from build123d import *

# Parameters (mm, degrees)
BOSS_EXTRUDE1_DEPTH = 5


with BuildPart() as part:
    # Sketch1 → Boss-Extrude1 (new body)
    with BuildSketch(Plane.XY):
        with BuildLine():
            Line((-150, 40), (-71.83, 40))
            Line((-71.83, 40), (-71.83, -40))
            Line((-71.83, -40), (-150, -40))
            Line((-150, -40), (-150, -100))
            ThreePointArc((-150, -100), (-147.071067812, -107.071067812), (-140, -110))
            Line((-140, -110), (140, -110))
            ThreePointArc((140, -110), (147.071067812, -107.071067812), (150, -100))
            Line((150, -100), (150, -40))
            Line((150, -40), (71.83, -40))
            Line((71.83, -40), (71.83, 40))
            Line((71.83, 40), (150, 40))
            Line((150, 40), (150, 100))
            ThreePointArc((150, 100), (147.071067812, 107.071067812), (140, 110))
            Line((140, 110), (-140, 110))
            ThreePointArc((-140, 110), (-147.071067812, 107.071067812), (-150, 100))
            Line((-150, 100), (-150, 40))
        make_face()
    extrude(amount=BOSS_EXTRUDE1_DEPTH)


solid = part.part
Verification items for the finished model (mm, model axes). Round coordinates to 2 decimals unless told otherwise and drop trailing zeros. Loops run counter-clockwise (first coordinate to the right, second up) from the corner with the lowest first, then second, coordinate; pieces in that order, holes last. Notation, with made-up numbers: (50, 77.25) - (90, 77.25) arc R35 cw to (90, 109.25) - close; hole circle Ø2 at (-39.5, 2.5). An arc over 180 degrees is marked (long way). Use a Markdown table: item, result. Add a question column.
1. Thickness scan on probe 1 along Y at (x, z) = (-135, 4.6); probe 2 along X at (y, z) = (-15, 4.3); probe 3 along X at (y, z) = (100.5, 2.85). Record the ranges inside material, lowest first. Write a range as [from, to].
2. Section check A-A, the plane z = 3.2. Record the boundary of the cut face in (x, y), plus the area to 3 significant figures.
3. Section check C-C, the plane y = 27.5. Record the boundary of the cut face in (x, z).
4. Section check B-B, the plane x = -108. Record the boundary of the cut face in (y, z), plus the area to 3 significant figures.
5. Gauge pin test, flat end, axial feed: pin 1 (2.5 mm diameter, centred on y = -7.5, z = 3, fed in from +X). Record the tip position at first contact, or that the pin passes through.
Checks:
| question | item | result |
|---|---|---|
| 1 | probe 1 | y = [-110, -40], [40, 110] |
| 1 | probe 2 | x = [-71.83, 71.83] |
| 1 | probe 3 | x = [-149.99, 149.99] |
| 2 | outline | (-150, -100) arc R10 ccw to (-140, -110) - (140, -110) arc R10 ccw to (150, -100) - (150, -40) - (71.83, -40) - (71.83, 40) - (150, 40) - (150, 100) arc R10 ccw to (140, 110) - (-140, 110) arc R10 ccw to (-150, 100) - (-150, 40) - (-71.83, 40) - (-71.83, -40) - (-150, -40) - close |
| 2 | area | 53,400 mm^2 |
| 3 | outline | (-71.83, 0) - (71.83, 0) - (71.83, 5) - (-71.83, 5) - close |
| 4 | outline | (-110, 0) - (-40, 0) - (-40, 5) - (-110, 5) - close; (40, 0) - (110, 0) - (110, 5) - (40, 5) - close |
| 4 | area | 700 mm^2 |
| 5 | pin 1 | stops at x = 71.83 |
